Design review of the part built by this model. Coordinates are the model's own, in mm. Face numbers are marked on the shaded views. A direction names the side the tool comes from. Coordinates: 2 decimals unless noted, no trailing zeros. Write each loop counter-clockwise with the first axis right and the second up, starting at its lowest first coordinate (ties: lowest second). Pieces come first, ordered by that corner, then holes. Notation, with made-up numbers: (44.25, -22) - (49.25, -22) arc R18 cw to (49.25, -10) - close; hole circle Ø6 at (53, 89). An arc over 180 degrees is marked (long way). One line per item, written item: value.
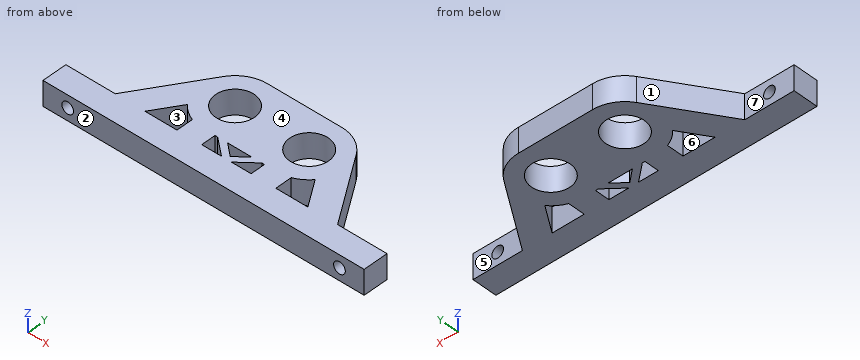
from build123d import *

# Parameters (mm, degrees)
BOSS_EXTRUDE1_DEPTH = 6.35
SKETCH2_R           = 5
CUT_EXTRUDE1_DEPTH  = 55.624765446
SKETCH3_R           = 1.5
CUT_EXTRUDE2_DEPTH  = 56.60442878


with BuildPart() as part:
    # Sketch1 → Boss-Extrude1 (new body)
    with BuildSketch(Plane.XY):
        with BuildLine():
            Line((19.05, 9), (0, 9))
            ThreePointArc((0, 9), (-4.283191939, 7.915444827), (-7.534082106, 4.923170403))
            Line((-7.534082106, 4.923170403), (-19.05, -12.7))
            Line((-19.05, -12.7), (-31.75, -12.7))
            Line((-31.75, -12.7), (-31.75, -19.05))
            Line((-31.75, -19.05), (50.8, -19.05))
            Line((50.8, -19.05), (50.8, -12.7))
            Line((50.8, -12.7), (38.1, -12.7))
            Line((38.1, -12.7), (26.584082106, 4.923170403))
            ThreePointArc((26.584082106, 4.923170403), (23.333191939, 7.915444827), (19.05, 9))
        make_face()
        Polygon((3.862011, -9), (8.255, -12.7), (3.175, -12.7), (3.175, -9), align=None, mode=Mode.SUBTRACT)
        Polygon((12.647989, -9), (9.525, -11.63034105), (6.402011, -9), (9.525, -9), align=None, mode=Mode.SUBTRACT)
        with BuildLine():
            Line((30.458149598, -12.7), (22.225, -12.7))
            Line((22.225, -12.7), (22.225, -8.421364201))
            ThreePointArc((22.225, -8.421364201), (24.252671243, -7.343855386), (25.941688674, -5.788318169))
            Line((25.941688674, -5.788318169), (30.458149598, -12.7))
        make_face(mode=Mode.SUBTRACT)
        Polygon((15.875, -12.7), (10.795, -12.7), (15.187989, -9), (15.875, -9), align=None, mode=Mode.SUBTRACT)
        with BuildLine():
            ThreePointArc((-6.891688674, -5.788318169), (-5.202671243, -7.343855386), (-3.175, -8.421364201))
            Line((-3.175, -8.421364201), (-3.175, -12.7))
            Line((-3.175, -12.7), (-11.408149598, -12.7))
            Line((-11.408149598, -12.7), (-6.891688674, -5.788318169))
        make_face(mode=Mode.SUBTRACT)
    extrude(amount=-BOSS_EXTRUDE1_DEPTH)

    # Sketch2 → Cut-Extrude1 (cut, through all)
    with BuildSketch(Plane.XY):
        Circle(SKETCH2_R)
        with Locations((19.05, 0)):
            Circle(SKETCH2_R)
    extrude(amount=-CUT_EXTRUDE1_DEPTH, mode=Mode.SUBTRACT)

    # Sketch3 → Cut-Extrude2 (cut, through all)
    with BuildSketch(Plane(origin=(0, -12.7, 0), x_dir=(1, 0, 0), z_dir=(0, 1, 0))):
        with Locations(Location((44.45, 3.175, 0), (0, 0, 270))):
            Circle(SKETCH3_R)
        with Locations(Location((-25.4, 3.175, 0), (0, 0, 270))):
            Circle(SKETCH3_R)
    extrude(amount=-CUT_EXTRUDE2_DEPTH, mode=Mode.SUBTRACT)


solid = part.part
1. Wall thickness on line 1 along X through (y, z) = (-13.75, -3); line 2 along Y through (x, z) = (0, -3); line 3 along X through (y, z) = (0.75, -2.25): over which ranges is each line inside the solid? List them lowest first.
Answer block:
line 1: x = -31.75 to -26.89, -23.91 to 42.96, 45.94 to 50.8
line 2: y = -19.05 to -5, 5 to 9
line 3: x = -10.26 to -4.94, 4.94 to 14.11, 23.99 to 29.31
2. Insertion check: pin 1 Ø1.5 at (x, z) = (41.5, -3.5) entering from +Y; pin 2 Ø2 at (y, z) = (5.5, -2.5) entering from +X; pin 3 Ø1.8 at (y, z) = (-11.5, -2.5) entering from +X. Each pin has a flat end and moves straight along its axis. Give the tip position at first contact, or say it passes through.
Answer block:
pin 1: stops at y = -12.7
pin 2: stops at x = 26.86
pin 3: stops at x = 37.9
3. Consider section C-C, the plane z = -2.5. Give the number of separate pieces and of enclosed holes in the cut face, then the cut area to 3 significant figures.
Answer block:
separate pieces: 3
enclosed holes: 7
area: 1,160 mm^2
4. For the marked faces 4, 5, 6 and 7, list the 3-axis set-ups (+Z, -Z, +X, -X, +Y, -Y) from which the entire face can be reached by the end or side of a thin tool; tool diameter is ignored.
Answer block:
face 4: +Z, +X, -X, +Y, -Y
face 5: +Z, -Z, +X, +Y
face 6: +Z, -Z
face 7: +Z, -Z, -X, +Y
5. Mouldability with a two-part tool opening along Y and no side actions: class the marked faces 1, 2 and 3 as released by +Y, released by -Y, zero draft, split by the parting line, or undercut.
Answer block:
face 1: released by +Y
face 2: released by -Y
face 3: undercut
6. Consider section A-A, the plane x = 44.45. Write out the cut boundary in (y, z) (3 decimals).
Answer block:
outline: (-19.05, -6.35) - (-12.7, -6.35) - (-12.7, -4.675) - (-19.05, -4.675) - close; (-19.05, -1.675) - (-12.7, -1.675) - (-12.7, 0) - (-19.05, 0) - close
7. Consider section B-B, the plane y = -1.75. Write out the cut boundary in (x, z).
Answer block:
outline: (-11.89, -6.35) - (-4.68, -6.35) - (-4.68, 0) - (-11.89, 0) - close; (4.68, -6.35) - (14.37, -6.35) - (14.37, 0) - (4.68, 0) - close; (23.73, -6.35) - (30.94, -6.35) - (30.94, 0) - (23.73, 0) - close
8. Consider section D-D, the plane y = 3.5. Write out the cut boundary in (x, z).
Answer block:
outline: (-8.46, -6.35) - (-3.57, -6.35) - (-3.57, 0) - (-8.46, 0) - close; (3.57, -6.35) - (15.48, -6.35) - (15.48, 0) - (3.57, 0) - close; (22.62, -6.35) - (27.51, -6.35) - (27.51, 0) - (22.62, 0) - close
